Drawing for the job (mm, zero at the part's lowest x, y, z). A direction names the side the tool comes from. Give positions to 0.01 mm unless a question says otherwise; leave off trailing zeros. Order: outer loops, then holes, each group sorted by start corner. A loop starts at its lowest first (then second) coordinate and runs counter-clockwise, first axis right, second up. Notation, with made-up numbers: (-35.5, -14.75) - (4.5, -14.75) arc R19 ccw to (4.5, 9.25) - close; hole circle Ø8 at (17, -34). An arc over 180 degrees is marked (long way). One line per item, written item: value.
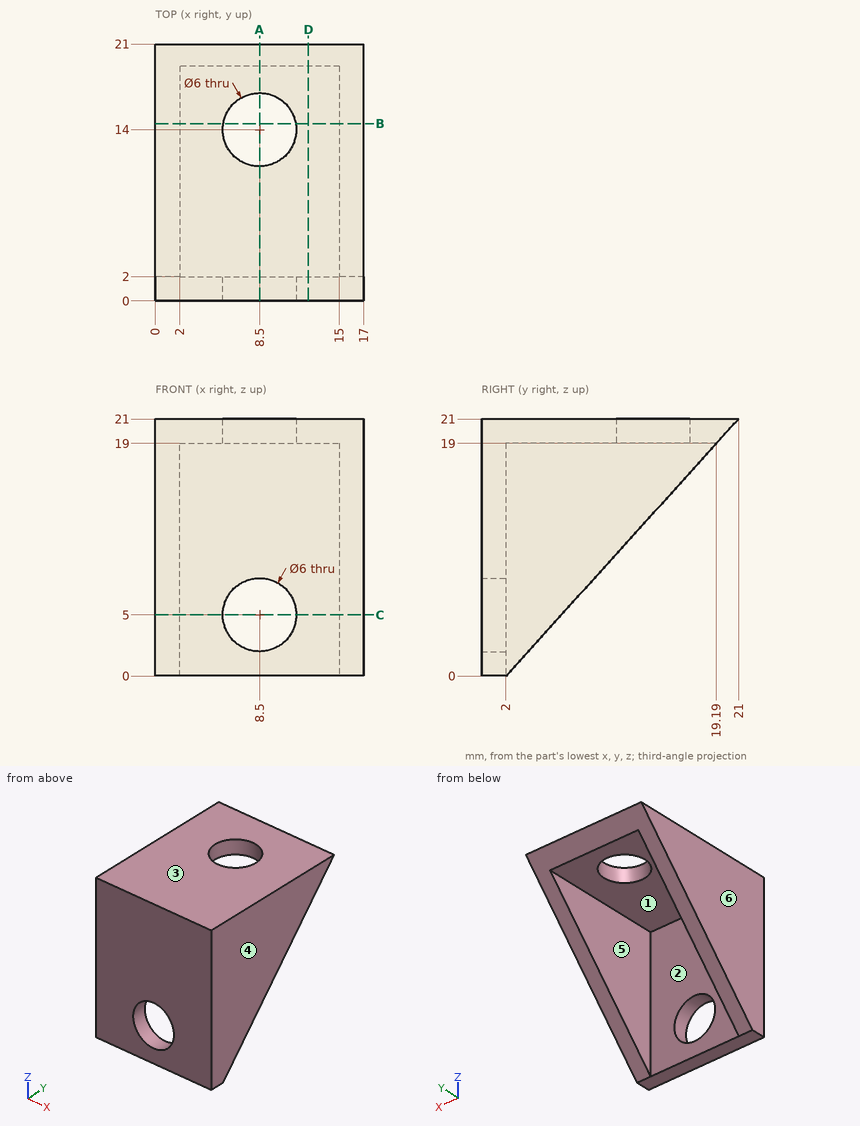
1) Pin check, flat tips, straight feed: pin 1 (6 mm diameter, centred on x = 6, y = 5.5, fed in from -Z); pin 2 (6 mm diameter, centred on x = 6.5, z = 6.5, fed in from +Y). Stop position of each tip, or through.
Outcome:
pin 1: stops at z = 19
pin 2: stops at y = 2
2) Mould opens along X. For the marked faces 1, 2, 3 and 4 say: released by +X, released by -X, zero draft, split by the parting line, or undercut.
Outcome:
face 1: undercut
face 2: undercut
face 3: zero draft
face 4: released by +X
3) Cut at B-B, the plane y = 14.5. Give the cut face in (x, z) (1 decimal).
Outcome:
outline: (0, 13.8) - (2, 13.8) - (2, 19) - (5.5, 19) - (5.5, 21) - (0, 21) - close; (11.5, 19) - (15, 19) - (15, 13.8) - (17, 13.8) - (17, 21) - (11.5, 21) - close
4) Cut at D-D, the plane x = 12.5. Give the cut face in (y, z).
Outcome:
outline: (0, 0) - (2, 0) - (2, 19) - (19.19, 19) - (21, 21) - (0, 21) - close
5) Which spindle directions (+Z, -Z, +X, -X, +Y, -Y) get a long thin tool onto all of the face, cutting with end or side? Do the marked faces 5 and 6. Say none if no direction does.
Outcome:
face 5: -Z, +Y
face 6: +Z, -Z, -X, +Y, -Y
6) Cut at A-A, the plane x = 8.5. Give the cut face in (y, z).
Outcome:
outline: (0, 0) - (2, 0) - (2, 2) - (0, 2) - close; (0, 8) - (2, 8) - (2, 19) - (11, 19) - (11, 21) - (0, 21) - close; (17, 19) - (19.19, 19) - (21, 21) - (17, 21) - close
7) Drill centre lines: line 1 along Z through (x, y) = (8.5, 0.8); line 2 along X through (y, z) = (2.5, 12.75); line 3 along Z through (x, y) = (2.5, 12.25). Where is each one in solid material? Low to high. Write a range as from..to.
Outcome:
line 1: z = 0..2, 8..21
line 2: x = 0..2, 15..17
line 3: z = 19..21
8) Cut at C-C, the plane z = 5. Give the cut face in (x, y).
Outcome:
outline: (0, 0) - (5.5, 0) - (5.5, 2) - (2, 2) - (2, 6.52) - (0, 6.52) - close; (11.5, 0) - (17, 0) - (17, 6.52) - (15, 6.52) - (15, 2) - (11.5, 2) - close
